Verification items for the finished model (mm, model axes). Give positions to 0.01 mm unless a question says otherwise; leave off trailing zeros. Loops run counter-clockwise (first coordinate to the right, second up) from the corner with the lowest first, then second, coordinate; pieces in that order, holes last. Notation, with made-up numbers: (69.5, 85.25) - (96.5, 85.25) arc R18 ccw to (96.5, 90.25) - close; hole circle Ø2 at (66.25, 22). An arc over 180 degrees is marked (long way). Answer in a Markdown table with one row per item.
```python
from build123d import *

# Parameters (mm, degrees)
EXTRUDE_1_DEPTH     = 55.63
SKETCH_2_R          = 1.25
CUT_EXTRUDE_1_DEPTH = 55.63
EXTRUDE_START       = 4.490261
SKETCH_3_R          = 1.25
EXTRUDE_2_DEPTH     = 4.490261


with BuildPart() as part:
    # 草图1 → 凸台-拉伸1 (new body)
    with BuildSketch(Plane(origin=(0, 0, 0), x_dir=(1, 0, 0), z_dir=(0, 1, 0))):
        Polygon((0.940938815, -1.454178169), (1.729824643, 0.087787833), (0.788885828, 1.541966002), (-0.940938815, 1.454178169), (-1.729824643, -0.087787833), (-0.788885828, -1.541966002), align=None)
    extrude(amount=EXTRUDE_1_DEPTH)

    # 草图2 → 切除-拉伸1 (cut)
    with BuildSketch(Plane(origin=(0, 55.63, 0), x_dir=(1, 0, 0), z_dir=(0, 1, 0))):
        with Locations(Location((0, 0, 0), (0, 0, 270))):
            Circle(SKETCH_2_R)
    extrude(amount=-CUT_EXTRUDE_1_DEPTH, mode=Mode.SUBTRACT)

    # 草图3 → 凸台-拉伸2 (add)
    with BuildSketch(Plane(origin=(0, 55.63, 0), x_dir=(1, 0, 0), z_dir=(0, 1, 0)).offset(EXTRUDE_START)):
        Polygon((0.788885828, 1.541966002), (-0.940938815, 1.454178169), (-1.729824643, -0.087787833), (-0.788885828, -1.541966002), (0.940938815, -1.454178169), (1.729824643, 0.087787833), align=None)
        with Locations(Location((0, 0, 0), (0, 0, 270))):
            Circle(SKETCH_3_R, mode=Mode.SUBTRACT)
    extrude(amount=-EXTRUDE_2_DEPTH)


solid = part.part
```
Q1. Sectioned sample at A-A (x = 0). Record the cut outline in (y, z), and give its area (3 significant figures).
Completed:
| item | result |
|---|---|
| outline | (0, -1.5) - (60.12, -1.5) - (60.12, -1.25) - (0, -1.25) - close; (0, 1.25) - (60.12, 1.25) - (60.12, 1.5) - (0, 1.5) - close |
| area | 30.3 mm^2 |
Q2. Draft check along X on faces 1 (the face through (-1.22, 30.48, -0.27)), 2 (the face through (-1.27, 30.48, 0.8)), 3 (the face through (1, 0, 1)). Enter one of: +X half, -X half, draft (parallel to the pull), parting line (faces both ways), or undercut.
Completed:
| item | result |
|---|---|
| face 1 | undercut |
| face 2 | -X half |
| face 3 | draft |
Q3. Sectioned sample at B-B (y = 15). Record the cut outline in (x, z), and give its area (3 significant figures).
Completed:
| item | result |
|---|---|
| outline | (-1.73, 0.09) - (-0.94, -1.45) - (0.79, -1.54) - (1.73, -0.09) - (0.94, 1.45) - (-0.79, 1.54) - close; hole circle Ø2.5 at (0, 0) |
| area | 2.89 mm^2 |
Q4. Go/stop test with flat-tipped pins: P1, Ø1, axis at x = 0, y = 43, coming from the -Z side; P2, Ø1.5, axis at x = -0.5, y = 54, coming from the +Z side. Record where each tip stops, or that it passes through.
Completed:
| item | result |
|---|---|
| P1 | z = -1.53 |
| P2 | z = 1.54 |
Q5. Thickness scan on line 1 (X direction, y = 34.5, z = 0); line 2 (Z direction, x = 0.45, y = 51.5); line 3 (X direction, y = 57.5, z = 0.6). Record the ranges inside material, lowest first.
Completed:
| item | result |
|---|---|
| line 1 | -1.68 to -1.25, 1.25 to 1.68 |
| line 2 | -1.52 to -1.17, 1.17 to 1.48 |
| line 3 | -1.4 to -1.1, 1.1 to 1.38 |
